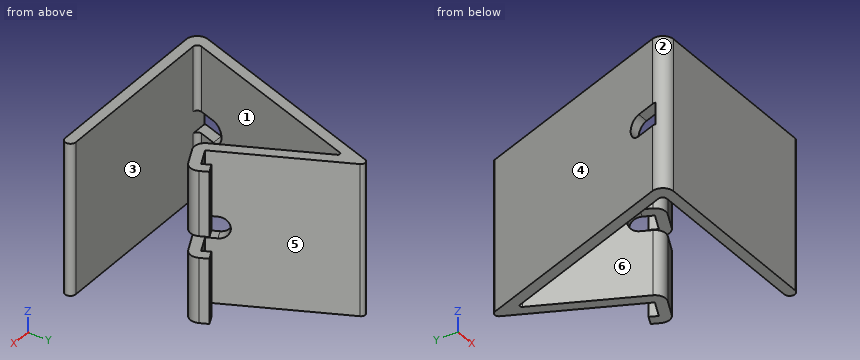
```python
from build123d import *

# Parameters (mm, degrees)
BOSS_EXTRUDE1_DEPTH     = 70
CUT_EXTRUDE2_DEPTH      = 40
CUT_EXTRUDE2_DEPTH_BACK = 40
CUT_EXTRUDE4_DEPTH      = 20


with BuildPart() as part:
    # Sketch1 → Boss-Extrude1 (new body)
    with BuildSketch(Plane.XY):
        with BuildLine():
            ThreePointArc((7.140740034, 0), (3.044979812, 2.132117818), (2.44227693, 6.710100717))
            Line((2.44227693, 6.710100717), (37.680897145, 103.527414051))
            ThreePointArc((37.680897145, 103.527414051), (39.473043612, 104.841470208), (41.372897961, 103.688610288))
            Line((41.372897961, 103.688610288), (66.802503496, 49.154645233))
            Line((66.802503496, 49.154645233), (75.412427472, 53.16951872))
            Line((75.412427472, 53.16951872), (73.721954425, 56.794749868))
            Line((73.721954425, 56.794749868), (78.253493361, 58.907841176))
            Line((78.253493361, 58.907841176), (79.943966408, 55.282610028))
            ThreePointArc((79.943966408, 55.282610028), (80.110890576, 51.459418003), (77.525518781, 48.637979784))
            Line((77.525518781, 48.637979784), (68.915594804, 44.623106298))
            ThreePointArc((68.915594804, 44.623106298), (65.092402779, 44.456182129), (62.27096456, 47.041553924))
            Line((62.27096456, 47.041553924), (40.922521982, 92.823436775))
            ThreePointArc((40.922521982, 92.823436775), (39.972594808, 93.399866735), (39.076521575, 92.742838656))
            Line((39.076521575, 92.742838656), (8.117650806, 7.684040287))
            ThreePointArc((8.117650806, 7.684040287), (8.358731959, 5.852847127), (9.997036047, 5))
            Line((9.997036047, 5), (90, 5))
            ThreePointArc((90, 5), (92.5, 2.5), (90, 0))
            Line((90, 0), (7.140740034, 0))
        make_face()
    extrude(amount=-BOSS_EXTRUDE1_DEPTH)

    # Sketch2 → Cut-Extrude2 (cut, two sides: drawn at the far end of the back side and taken through both)
    with BuildSketch(Plane(origin=(73.698483936, 34.366167454, 0), x_dir=(0, 0, -1), z_dir=(0.9063077870366539, 0.422618261740691, 0)).offset(-CUT_EXTRUDE2_DEPTH_BACK)):
        with BuildLine():
            Line((40, 16.317279836), (40, 21.317279836))
            ThreePointArc((40, 21.317279836), (35, 26.317279836), (30, 21.317279836))
            Line((30, 21.317279836), (30, 16.317279836))
            Line((30, 16.317279836), (30, 11.317279836))
            Line((30, 11.317279836), (40, 11.317279836))
            Line((40, 11.317279836), (40, 16.317279836))
        make_face()
    extrude(amount=CUT_EXTRUDE2_DEPTH + CUT_EXTRUDE2_DEPTH_BACK, mode=Mode.SUBTRACT)

    # Sketch5 → Cut-Extrude4 (cut)
    with BuildSketch(Plane(origin=(0, 0, 0), x_dir=(0, 0, -1), z_dir=(1, 0, 0))):
        with BuildLine():
            Line((40, 10), (40, 15))
            ThreePointArc((40, 15), (35, 20), (30, 15))
            Line((30, 15), (30, 10))
            Line((30, 10), (30, 5))
            Line((30, 5), (40, 5))
            Line((40, 5), (40, 10))
        make_face()
    extrude(amount=CUT_EXTRUDE4_DEPTH, mode=Mode.SUBTRACT)


solid = part.part
```
For this review, take the finished solid that the model builds, in its own axes (mm). Face numbers are marked on the shaded views. A direction names the side the tool comes from. Give positions to 0.01 mm unless a question says otherwise; leave off trailing zeros. Order: outer loops, then holes, each group sorted by start corner. A loop starts at its lowest first (then second) coordinate and runs counter-clockwise, first axis right, second up.
1) Take a section at A-A (z = -37.5). Give the boundary of the cut face in (x, y).
2) Take a section at D-D (z = -6). Give the boundary of the cut face in (x, y), then the cut area to 3 significant figures.
3) The part is to be moulded in two halves that separate along X. For the marked faces 1, 2 and 3, say which applies: released by +X, released by -X, zero draft, split by the parting line, or undercut.
4) Take a section at B-B (x = 27.5). Give the boundary of the cut face in (y, z).
5) Take a section at C-C (y = 67). Give the boundary of the cut face in (x, z).
6) For the marked faces 4, 5 and 6, list the 3-axis set-ups (+Z, -Z, +X, -X, +Y, -Y) from which the entire face can be reached by the end or side of a thin tool; tool diameter is ignored.
7) Insertion check: pin 1 (10 mm diameter, centred on y = 55, z = -48, fed in from +X); pin 2 (1 mm diameter, centred on x = 75.5, z = -56, fed in from +Y); pin 3 (8 mm diameter, centred on x = 69.5, y = 11, fed in from +Z). Each pin has a flat end and moves straight along its axis. Give the tip position at first contact, or say it passes through.
8) Wall thickness on line 1 (Z direction, x = 67, y = 46); line 2 (Y direction, x = 88, z = -56.5); line 3 (X direction, y = 75, z = -32.5): over which ranges is each line inside the solid? List them lowest first.
Derived:
1. outline: (2.14, 5) arc R5 ccw to (7.14, 0) - (90, 0) arc R2.5 ccw to (90, 5) - close; (7.04, 19.33) - (12.36, 19.33) - (39.08, 92.74) arc R1 cw to (40.92, 92.82) - (58.33, 55.5) - (62.86, 57.61) - (41.37, 103.69) arc R2 ccw to (37.68, 103.53) - close
2. outline: (2.44, 6.71) arc R5 ccw to (7.14, 0) - (90, 0) arc R2.5 ccw to (90, 5) - (10, 5) arc R2 cw to (8.12, 7.68) - (39.08, 92.74) arc R1 cw to (40.92, 92.82) - (62.27, 47.04) arc R5 ccw to (68.92, 44.62) - (77.53, 48.64) arc R5 ccw to (79.94, 55.28) - (78.25, 58.91) - (73.72, 56.79) - (75.41, 53.17) - (66.8, 49.15) - (41.37, 103.69) arc R2 ccw to (37.68, 103.53) - close
2. area: 1,360 mm2
3. face 1: undercut
3. face 2: released by -X
3. face 3: zero draft
4. outline: (0, -70) - (5, -70) - (5, 0) - (0, 0) - close; (60.94, -70) - (75.56, -70) - (75.56, 0) - (60.94, 0) - close
5. outline: (24.39, -70) - (29.71, -70) - (29.71, 0) - (24.39, 0) - close; (52.96, -70) - (58.48, -70) - (58.48, 0) - (52.96, 0) - close
6. face 4: +Z, -Z, -X, +Y
6. face 5: +Z, -Z, +Y
6. face 6: +Z, -Z
7. pin 1: stops at x = 80.41
7. pin 2: stops at y = 57.86
7. pin 3: passes through
8. line 1: z = -70 to -40, -30 to 0
8. line 2: y = 0 to 5
8. line 3: x = 27.3 to 32.62, 49.23 to 54.75
